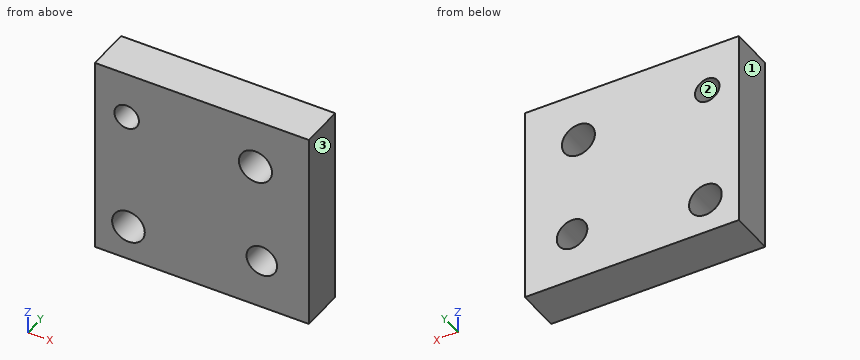
from build123d import *

# Parameters (mm, degrees)
F0_W     = 48.529239
F0_H     = 45.212935
F0_R     = 3.705071
F0_R_2   = 3.464323
F0_R_3   = 2.775839
F0_R_4   = 3.746018
F1_DEPTH = 10


with BuildPart() as f1:
    # F0 (on Front) → F1 (new body)
    with BuildSketch(Plane.XZ):
        with Locations((-1.263026, -5.951959)):
            Rectangle(F0_W, F0_H)
        with Locations((-17.919248, -20.630553)):
            Circle(F0_R, mode=Mode.SUBTRACT)
        with Locations((12.308709, -17.250935)):
            Circle(F0_R_2, mode=Mode.SUBTRACT)
        with Locations((-18.330511, 6.188568)):
            Circle(F0_R_3, mode=Mode.SUBTRACT)
        with Locations((10.869283, 5.364367)):
            Circle(F0_R_4, mode=Mode.SUBTRACT)
    extrude(amount=F1_DEPTH)


solid = f1.part
Could you check a few things on this model? Use its own coordinates, in mm. Face numbers are marked on the shaded views. Coordinates: 2 decimals unless noted, no trailing zeros. Loops run counter-clockwise (first coordinate to the right, second up) from the corner with the lowest first, then second, coordinate; pieces in that order, holes last.
1. We'd pull the mould along X, two halves only. Please class the marked faces 1, 2 and 3: released by +X, released by -X, zero draft, split by the parting line, or undercut.
2. Imagine slicing it at B-B (x = 13). Please give me the cut outline in (y, z).
3. Imagine slicing it at C-C (y = -0.75). Please give me the cut outline in (x, z).
4. Imagine slicing it at D-D (z = -23.5). Please give me the cut outline in (x, y), and give its area (3 significant figures).
5. I need wall thicknesses on L1, parallel to Z at x = -17, y = -1.5; L2, parallel to Z at x = 10.5, y = -6.25; L3, parallel to X at y = -5.25, z = 4. Which ranges of each line are inside material? Lowest first, please.
6. Imagine slicing it at A-A (z = 2.5). Please give me the cut outline in (x, y), and give its area (3 significant figures).
Computed values:
1. face 1: released by -X
1. face 2: undercut
1. face 3: released by +X
2. outline: (-10, -28.56) - (0, -28.56) - (0, -20.65) - (-10, -20.65) - close; (-10, -13.86) - (0, -13.86) - (0, 2.28) - (-10, 2.28) - close; (-10, 8.45) - (0, 8.45) - (0, 16.65) - (-10, 16.65) - close
3. outline: (-25.53, -28.56) - (23, -28.56) - (23, 16.65) - (-25.53, 16.65) - close; hole circle Ø7.41 at (-17.92, -20.63); hole circle Ø5.55 at (-18.33, 6.19); hole circle Ø7.49 at (10.87, 5.36); hole circle Ø6.93 at (12.31, -17.25)
4. outline: (-25.53, -10) - (-20.26, -10) - (-20.26, 0) - (-25.53, 0) - close; (-15.58, -10) - (23, -10) - (23, 0) - (-15.58, 0) - close
4. area: 438 mm2
5. L1: z = -28.56 to -24.22, -17.04 to 3.75, 8.62 to 16.65
5. L2: z = -28.56 to -20.21, -14.3 to 1.64, 9.09 to 16.65
5. L3: x = -25.53 to -20.04, -16.62 to 7.38, 14.36 to 23
6. outline: (-25.53, -10) - (8.46, -10) - (8.46, 0) - (-25.53, 0) - close; (13.28, -10) - (23, -10) - (23, 0) - (13.28, 0) - close
6. area: 437 mm2
